Input: part model. Units: mm. Frame: model coordinates. Give positions to 0.01 mm unless a question says otherwise; leave off trailing zeros. Order: outer loops, then holes, each group sorted by start corner. A loop starts at its lowest first (then second) coordinate and runs counter-clockwise, first axis right, second up.
```python
from build123d import *

# Parameters (mm, degrees)
F0_R     = 19.05
F1_DEPTH = 50.8
F2_R     = 9.525
F3_DEPTH = 25.4
F4_SIZE  = 1.524
F5_SIZE  = 1.524
F6_SIZE  = 1.524
F7_R     = 5.08
F8_R     = 5.08


with BuildPart() as f1:
    # F0 (on Front) → F1 (new body)
    with BuildSketch(Plane.XZ):
        with BuildLine():
            Line((35.921024, -38.1), (35.921024, 12.7))
            ThreePointArc((35.921024, 12.7), (0, 38.034383), (-35.921024, 12.7))
            Line((-35.921024, 12.7), (-35.921024, -38.1))
            Line((-35.921024, -38.1), (35.921024, -38.1))
        make_face()
        Circle(F0_R, mode=Mode.SUBTRACT)
    extrude(amount=F1_DEPTH)

    # F2 (on face) → F3 (cut)
    with BuildSketch(Plane(origin=(0, 0, -38.1), x_dir=(1, 0, 0), z_dir=(0, 0, -1))):
        with Locations((0, 25.4)):
            Circle(F2_R)
    extrude(amount=-F3_DEPTH, mode=Mode.SUBTRACT)

    # F4
    f4_edges = [f1.edges().sort_by_distance(p)[0] for p in [
        (0, -50.8, 38.034383),
        (-35.921024, -50.8, -12.7),
        (0, -50.8, -38.1),
        (35.921024, -50.8, -12.7),
        (-19.05, -50.8, 0),
    ]]
    chamfer(f4_edges, length=F4_SIZE)

    # F5
    f5_edges = [f1.edges().sort_by_distance(p)[0] for p in [
        (0, 0, 38.034383),
        (35.921024, 0, -12.7),
        (0, 0, -38.1),
        (-35.921024, 0, -12.7),
        (-19.05, 0, 0),
    ]]
    chamfer(f5_edges, length=F5_SIZE)

    # F6
    f6_edges = [f1.edges().sort_by_distance(p)[0] for p in [
        (35.921024, -25.4, -38.1),
        (-35.921024, -25.4, -38.1),
        (-9.525, -25.4, -38.1),
    ]]
    chamfer(f6_edges, length=F6_SIZE)

    # F7
    f7_edges = [f1.edges().sort_by_distance(p)[0] for p in [
        (-35.921024, -25.4, 12.7),
    ]]
    fillet(f7_edges, radius=F7_R)

    # F8
    f8_edges = [f1.edges().sort_by_distance(p)[0] for p in [
        (35.921024, -25.4, 12.7),
    ]]
    fillet(f8_edges, radius=F8_R)


solid = f1.part
```
1) Line query: probe 1 along Y at (x, z) = (0, -30) (3 decimals); probe 2 along X at (y, z) = (-25.4, -26.25) (3 decimals); probe 3 along X at (y, z) = (-33, -5). Output: solid intervals per line, ascending.
2) First-contact query: P1, Ø4, axis at x = -1.5, y = -15.5, coming from the +Z side; P2, Ø2, axis at x = -11, z = -25, coming from the +Y side; P3, Ø8, axis at x = -26.5, y = -15, coming from the +Z side; P4, Ø1.5, axis at x = 22.5, y = -22, coming from the +Z side. Flat tips, straight axial feed; report the tip coordinate or a pass-through.
3) Cut plane D-D (z = 0). Return the cut outline in (x, y).
4) Cut plane C-C (y = -25.4). Return the cut outline in (x, z) (3 decimals), then the cut area to 3 significant figures.
5) Pull-direction query (Y, two-part tool) for faces 1 (the face through (0.634, -50.557, 36.748)), 2 (the face through (-9.516, -25.819, -26.677)), 3 (the face through (7, -36, -38.1)); classes: pulls with the +Y half, pulls with the -Y half, needs draft (parallel to the pull), parting line crosses it, or undercut.
6) Cut plane A-A (z = -31). Return the cut outline in (x, y) (3 decimals).
7) Cut plane B-B (x = 0). Return the cut outline in (y, z) (3 decimals), then the cut area to 3 significant figures.
Geometry says:
1. probe 1: y = -50.8 to -34.925, -15.875 to 0
1. probe 2: x = -35.921 to -9.525, 9.525 to 35.921
1. probe 3: x = -35.92 to -18.38, 18.38 to 35.92
2. P1: stops at z = 38.03
2. P2: stops at y = 0
2. P3: stops at z = 30.69
2. P4: stops at z = 31.22
3. outline: (-35.92, -49.28) - (-34.4, -50.8) - (-20.57, -50.8) - (-19.05, -49.28) - (-19.05, -1.52) - (-20.57, 0) - (-34.4, 0) - (-35.92, -1.52) - close; (19.05, -49.28) - (20.57, -50.8) - (34.4, -50.8) - (35.92, -49.28) - (35.92, -1.52) - (34.4, 0) - (20.57, 0) - (19.05, -1.52) - close
4. outline: (-35.921, -36.576) - (-34.397, -38.1) - (-11.049, -38.1) - (-9.525, -36.576) - (-9.525, -16.498) arc R19.05 cw (long way) to (9.525, -16.498) - (9.525, -36.576) - (11.049, -38.1) - (34.397, -38.1) - (35.921, -36.576) - (35.921, 11.79) arc R5.08 ccw to (35.581, 13.617) arc R38.133 ccw to (-35.581, 13.617) arc R5.08 ccw to (-35.921, 11.79) - close
4. area: 3,450 mm2
5. face 1: pulls with the -Y half
5. face 2: undercut
5. face 3: needs draft
6. outline: (-35.921, -49.276) - (-34.397, -50.8) - (34.397, -50.8) - (35.921, -49.276) - (35.921, -1.524) - (34.397, 0) - (-34.397, 0) - (-35.921, -1.524) - close; hole circle Ø19.05 at (0, -25.4)
7. outline: (-50.8, -36.576) - (-49.276, -38.1) - (-36.449, -38.1) - (-34.925, -36.576) - (-34.925, -19.05) - (-49.276, -19.05) - (-50.8, -20.574) - close; (-50.8, 20.574) - (-49.276, 19.05) - (-1.524, 19.05) - (0, 20.574) - (0, 36.51) - (-1.524, 38.034) - (-49.276, 38.034) - (-50.8, 36.51) - close; (-15.875, -36.576) - (-14.351, -38.1) - (-1.524, -38.1) - (0, -36.576) - (0, -20.574) - (-1.524, -19.05) - (-15.875, -19.05) - close
7. area: 1,560 mm2
